Verification items for the finished model (mm, model axes). A direction names the side the tool comes from. Round coordinates to 2 decimals unless told otherwise and drop trailing zeros. Loops run counter-clockwise (first coordinate to the right, second up) from the corner with the lowest first, then second, coordinate; pieces in that order, holes last. Notation, with made-up numbers: M 75,82.5 L 83,82.5 A9 ccw 83,99.5 Z; hole C -11,76 d6. An arc over 180 degrees is marked long. Answer as CSV lines item,"result".
```python
from build123d import *

# Parameters (mm, degrees)
SKETCH1_W           = 5
SKETCH1_H           = 110
SKETCH1_W_2         = 30
SKETCH1_H_2         = 20
BOSS_EXTRUDE1_DEPTH = 35
SKETCH9_W           = 10
SKETCH9_H           = 20
BOSS_EXTRUDE2_DEPTH = 70
RIB1_REACH          = 141.732
SKETCH10_WALL_W     = 372.705210204
SKETCH10_WALL_H     = 4
SKETCH11_W          = 5
SKETCH11_H          = 5
CUT_EXTRUDE2_DEPTH  = 10


with BuildPart() as part:
    # Sketch1 → Boss-Extrude1 (new, symmetric)
    with BuildSketch(Plane(origin=(0, 0, 0), x_dir=(0, 0, -1), z_dir=(1, 0, 0))):
        with Locations((-12.5, 65)):
            Rectangle(SKETCH1_W, SKETCH1_H)
        Rectangle(SKETCH1_W_2, SKETCH1_H_2)
    extrude(amount=BOSS_EXTRUDE1_DEPTH, both=True)

    # Sketch9 → Boss-Extrude2 (add, through all)
    with BuildSketch(Plane(origin=(35, 0, 0), x_dir=(0, 0, -1), z_dir=(1, 0, 0))):
        with Locations((-5, 110)):
            Rectangle(SKETCH9_W, SKETCH9_H)
    extrude(amount=-BOSS_EXTRUDE2_DEPTH)

    # Sketch10 wall → Rib1 (add, up to next)
    with BuildSketch(Plane(origin=(35, 55, -7.5), x_dir=(0, -0.986393923832, -0.164398987305), z_dir=(0, 0.164398987305, -0.986393923832)), mode=Mode.PRIVATE) as rib1_sk1:
        with Locations((0, 2)):
            Rectangle(SKETCH10_WALL_W, SKETCH10_WALL_H)
    rib1_tool1 = extrude(rib1_sk1.sketch, amount=-RIB1_REACH, mode=Mode.PRIVATE) - part.part
    rib1 = rib1_tool1.solids().sort_by_distance((35, 55, -7.5))[0]
    add(rib1)

    # Mirror1: Rib1 across plane
    add(rib1.mirror(Plane(origin=(0, 0, 0), x_dir=(0, 0, 1), z_dir=(1, 0, 0))))

    # Sketch11 → Cut-Extrude2 (cut)
    with BuildSketch(Plane.XY.offset(15)):
        with Locations((15, 111.5)):
            Rectangle(SKETCH11_W, SKETCH11_H)
        with Locations((-15, 111.5)):
            Rectangle(SKETCH11_W, SKETCH11_H)
    extrude(amount=-CUT_EXTRUDE2_DEPTH, mode=Mode.SUBTRACT)


solid = part.part
```
1) Set-up check for faces 5 (the flat face through (0, 110, 0)), 6 (the flat face through (-15, 109, 10)), 7 (the flat face through (0, 10, -2)): record each of +Z, -Z, +X, -X, +Y, -Y from which the full face is reachable in a straight line by a thin tool's end or side.
Here are the results:
face 5,"-Z, +X, -X, +Y"
face 6,"+Z"
face 7,"-Z"
2) Draft check along Y on faces 1 (the flat face through (31, 45, 0)), 2 (the flat face through (0, -10, 0)), 3 (the flat face through (-33, 55.6, -7.4)), 4 (the flat face through (-35, 41, 1)). Enter one of: +Y half, -Y half, draft (parallel to the pull), parting line (faces both ways), or undercut.
Here are the results:
face 1,"undercut"
face 2,"-Y half"
face 3,"+Y half"
face 4,"draft"
3) Go/stop test with flat-tipped pins: pin 1 (22 mm diameter, centred on x = 4.5, y = 109.5, fed in from -Z); pin 2 (8 mm diameter, centred on x = 14.5, z = -6.5, fed in from +Y); pin 3 (8 mm diameter, centred on x = -25.5, y = 52, fed in from -Z). Record where each tip stops, or that it passes through.
Here are the results:
pin 1,"stops at z = 0"
pin 2,"stops at y = 10"
pin 3,"stops at z = 10"
4) Section check C-C (y = 61). Record the cut outline in (x, z).
Here are the results:
outline,"M -35,-6.5 L -31,-6.5 L -31,10 L 31,10 L 31,-6.5 L 35,-6.5 L 35,15 L -35,15 Z"
5) Section check D-D (x = -22). Record the cut outline in (y, z), plus the area to 3 significant figures.
Here are the results:
outline,"M -10,-15 L 10,-15 L 10,10 L 100,10 L 100,0 L 120,0 L 120,15 L -10,15 Z"
area,"1,350 mm^2"
6) Section check A-A (z = 8). Record the cut outline in (x, y).
Here are the results:
outline,"M -35,-10 L 35,-10 L 35,120 L -35,120 Z; hole M -31,10 L 31,10 L 31,100 L -31,100 Z; hole M -17.5,109 L -12.5,109 L -12.5,114 L -17.5,114 Z; hole M 12.5,109 L 17.5,109 L 17.5,114 L 12.5,114 Z"
7) Material ranges on probe 1 along X at (y, z) = (15, -6); probe 2 along Y at (x, z) = (0.5, 8); probe 3 along Z at (x, y) = (-15.5, 97), recorded low to high.
Here are the results:
probe 1,"x = -35 to -31, 31 to 35"
probe 2,"y = -10 to 10, 100 to 120"
probe 3,"z = 10 to 15"
8) Section check B-B (z = 1.75). Record the cut outline in (x, y).
Here are the results:
outline,"M -35,-10 L 35,-10 L 35,120 L -35,120 Z; hole M -31,10 L 31,10 L 31,100 L -31,100 Z"
